Design review of the part built by this model. Coordinates are the model's own, in mm. Face numbers are marked on the shaded views. Round coordinates to 2 decimals unless told otherwise and drop trailing zeros. Use one line per item in the form item = value.
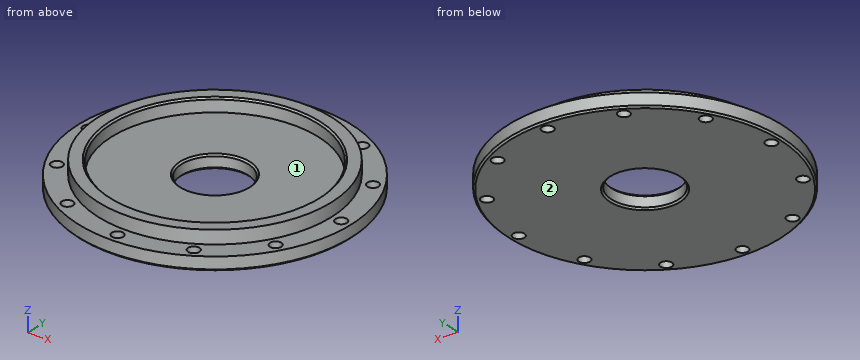
```python
from build123d import *

# Parameters (mm, degrees)
CUT_EXTRUDE_1_REACH = 60.121
SKETCH_2_R          = 1.7
CUT_EXTRUDE_2_REACH = 60.532
SKETCH_3_R          = 10
CHAMFER_1_SIZE      = 0.5


with BuildPart() as part:
    # 草图1 → 旋转1 (revolve)
    with BuildSketch(Plane(origin=(0, 0, 0), x_dir=(0, 0, -1), z_dir=(1, 0, 0)), mode=Mode.PRIVATE) as revolve_1_sk:
        Polygon((0, 0), (0, 41), (-4, 41), (-4, 35), (-8, 35), (-8, 31), (-4, 31), (-4, 0), align=None)
    revolve(revolve_1_sk.sketch.rotate(Axis((0, 0, 0), (0, 0, 1)), 90), axis=Axis((0, 0, 0), (0, 0, 1)))

    # 草图2 → 切除-拉伸1 (cut, up to next)
    with BuildSketch(Plane.XY.offset(4), mode=Mode.PRIVATE) as cut_extrude_1_sk1:
        with Locations((0, 38)):
            Circle(SKETCH_2_R)
    cut_extrude_1_tool1 = extrude(cut_extrude_1_sk1.sketch, amount=-CUT_EXTRUDE_1_REACH, mode=Mode.PRIVATE) & part.part
    # 草图2 → 切除-拉伸1 (cut, up to next)
    with BuildSketch(Plane.XY.offset(4), mode=Mode.PRIVATE) as cut_extrude_1_sk2:
        with Locations((19, 32.908965344)):
            Circle(SKETCH_2_R)
    cut_extrude_1_tool2 = extrude(cut_extrude_1_sk2.sketch, amount=-CUT_EXTRUDE_1_REACH, mode=Mode.PRIVATE) & part.part
    # 草图2 → 切除-拉伸1 (cut, up to next)
    with BuildSketch(Plane.XY.offset(4), mode=Mode.PRIVATE) as cut_extrude_1_sk3:
        with Locations((32.908965344, 19)):
            Circle(SKETCH_2_R)
    cut_extrude_1_tool3 = extrude(cut_extrude_1_sk3.sketch, amount=-CUT_EXTRUDE_1_REACH, mode=Mode.PRIVATE) & part.part
    # 草图2 → 切除-拉伸1 (cut, up to next)
    with BuildSketch(Plane.XY.offset(4), mode=Mode.PRIVATE) as cut_extrude_1_sk4:
        with Locations((38, 0)):
            Circle(SKETCH_2_R)
    cut_extrude_1_tool4 = extrude(cut_extrude_1_sk4.sketch, amount=-CUT_EXTRUDE_1_REACH, mode=Mode.PRIVATE) & part.part
    # 草图2 → 切除-拉伸1 (cut, up to next)
    with BuildSketch(Plane.XY.offset(4), mode=Mode.PRIVATE) as cut_extrude_1_sk5:
        with Locations((32.908965344, -19)):
            Circle(SKETCH_2_R)
    cut_extrude_1_tool5 = extrude(cut_extrude_1_sk5.sketch, amount=-CUT_EXTRUDE_1_REACH, mode=Mode.PRIVATE) & part.part
    # 草图2 → 切除-拉伸1 (cut, up to next)
    with BuildSketch(Plane.XY.offset(4), mode=Mode.PRIVATE) as cut_extrude_1_sk6:
        with Locations((19, -32.908965344)):
            Circle(SKETCH_2_R)
    cut_extrude_1_tool6 = extrude(cut_extrude_1_sk6.sketch, amount=-CUT_EXTRUDE_1_REACH, mode=Mode.PRIVATE) & part.part
    # 草图2 → 切除-拉伸1 (cut, up to next)
    with BuildSketch(Plane.XY.offset(4), mode=Mode.PRIVATE) as cut_extrude_1_sk7:
        with Locations((0, -38)):
            Circle(SKETCH_2_R)
    cut_extrude_1_tool7 = extrude(cut_extrude_1_sk7.sketch, amount=-CUT_EXTRUDE_1_REACH, mode=Mode.PRIVATE) & part.part
    # 草图2 → 切除-拉伸1 (cut, up to next)
    with BuildSketch(Plane.XY.offset(4), mode=Mode.PRIVATE) as cut_extrude_1_sk8:
        with Locations((-19, -32.908965344)):
            Circle(SKETCH_2_R)
    cut_extrude_1_tool8 = extrude(cut_extrude_1_sk8.sketch, amount=-CUT_EXTRUDE_1_REACH, mode=Mode.PRIVATE) & part.part
    # 草图2 → 切除-拉伸1 (cut, up to next)
    with BuildSketch(Plane.XY.offset(4), mode=Mode.PRIVATE) as cut_extrude_1_sk9:
        with Locations((-32.908965344, -19)):
            Circle(SKETCH_2_R)
    cut_extrude_1_tool9 = extrude(cut_extrude_1_sk9.sketch, amount=-CUT_EXTRUDE_1_REACH, mode=Mode.PRIVATE) & part.part
    # 草图2 → 切除-拉伸1 (cut, up to next)
    with BuildSketch(Plane.XY.offset(4), mode=Mode.PRIVATE) as cut_extrude_1_sk10:
        with Locations((-38, 0)):
            Circle(SKETCH_2_R)
    cut_extrude_1_tool10 = extrude(cut_extrude_1_sk10.sketch, amount=-CUT_EXTRUDE_1_REACH, mode=Mode.PRIVATE) & part.part
    # 草图2 → 切除-拉伸1 (cut, up to next)
    with BuildSketch(Plane.XY.offset(4), mode=Mode.PRIVATE) as cut_extrude_1_sk11:
        with Locations((-32.908965344, 19)):
            Circle(SKETCH_2_R)
    cut_extrude_1_tool11 = extrude(cut_extrude_1_sk11.sketch, amount=-CUT_EXTRUDE_1_REACH, mode=Mode.PRIVATE) & part.part
    # 草图2 → 切除-拉伸1 (cut, up to next)
    with BuildSketch(Plane.XY.offset(4), mode=Mode.PRIVATE) as cut_extrude_1_sk12:
        with Locations((-19, 32.908965344)):
            Circle(SKETCH_2_R)
    cut_extrude_1_tool12 = extrude(cut_extrude_1_sk12.sketch, amount=-CUT_EXTRUDE_1_REACH, mode=Mode.PRIVATE) & part.part
    add(cut_extrude_1_tool1.solids().sort_by_distance((0, 38, 4))[0], mode=Mode.SUBTRACT)
    add(cut_extrude_1_tool2.solids().sort_by_distance((19, 32.908965, 4))[0], mode=Mode.SUBTRACT)
    add(cut_extrude_1_tool3.solids().sort_by_distance((32.908965, 19, 4))[0], mode=Mode.SUBTRACT)
    add(cut_extrude_1_tool4.solids().sort_by_distance((38, 0, 4))[0], mode=Mode.SUBTRACT)
    add(cut_extrude_1_tool5.solids().sort_by_distance((32.908965, -19, 4))[0], mode=Mode.SUBTRACT)
    add(cut_extrude_1_tool6.solids().sort_by_distance((19, -32.908965, 4))[0], mode=Mode.SUBTRACT)
    add(cut_extrude_1_tool7.solids().sort_by_distance((0, -38, 4))[0], mode=Mode.SUBTRACT)
    add(cut_extrude_1_tool8.solids().sort_by_distance((-19, -32.908965, 4))[0], mode=Mode.SUBTRACT)
    add(cut_extrude_1_tool9.solids().sort_by_distance((-32.908965, -19, 4))[0], mode=Mode.SUBTRACT)
    add(cut_extrude_1_tool10.solids().sort_by_distance((-38, 0, 4))[0], mode=Mode.SUBTRACT)
    add(cut_extrude_1_tool11.solids().sort_by_distance((-32.908965, 19, 4))[0], mode=Mode.SUBTRACT)
    add(cut_extrude_1_tool12.solids().sort_by_distance((-19, 32.908965, 4))[0], mode=Mode.SUBTRACT)

    # 草图3 → 切除-拉伸2 (cut, up to next)
    with BuildSketch(Plane(origin=(0, 0, 0), x_dir=(-1, 0, 0), z_dir=(0, 0, -1)), mode=Mode.PRIVATE) as cut_extrude_2_sk1:
        Circle(SKETCH_3_R)
    cut_extrude_2_tool1 = extrude(cut_extrude_2_sk1.sketch, amount=-CUT_EXTRUDE_2_REACH, mode=Mode.PRIVATE) & part.part
    add(cut_extrude_2_tool1.solids().sort_by_distance((0, 0, 0))[0], mode=Mode.SUBTRACT)

    # 倒角1
    chamfer_1_edges = [part.edges().sort_by_distance(p)[0] for p in [
        (10, 0, 4),
        (10, 0, 0),
        (31, 0, 8),
        (41, 0, 0),
    ]]
    chamfer(chamfer_1_edges, length=CHAMFER_1_SIZE)


solid = part.part
```
Q1. To check wall thickness, follow line 1 along Y through (x, z) = (0, 5.05); line 2 along Y through (x, z) = (-19, 2.95); line 3 along Z through (x, y) = (-4.5, 37). State the ranges of each line that lie inside material, in increasing order. Write a range as from..to.
Calculated:
line_1 = -35..-31, 31..35
line_2 = -36.33..-34.61, -31.21..31.21, 34.61..36.33
line_3 = 0..4
Q2. For P1, Ø2.5, axis at x = 32.91, y = 19, coming from the -Z side; P2, Ø24.5, axis at x = 8, y = 2, coming from the +Z side; P3, Ø3, axis at y = -32, z = 3.5, coming from the +X side; P4, Ø1.5, axis at x = -11, z = 5.5, coming from the +Y side, all flat-tipped, find the tip position at first contact; note any pin that passes through.
Calculated:
P1 = through
P2 = 4
P3 = 27.4
P4 = 33.47
Q3. We need section A-A on x = 0. State how many separate pieces and enclosed holes the cut face has, then the cut area to 3 significant figures.
Calculated:
separate_pieces = 4
enclosed_holes = 0
area = 252 mm2
Q4. Draft analysis for pull direction Y (two halves, no side actions). For the marked faces 1 and 2, state which applies: released by +Y, released by -Y, zero draft, split by the parting line, or undercut.
Calculated:
face_1 = undercut
face_2 = zero draft
